from build123d import *

# Parameters (mm, degrees)
BOSS_EXTRUDE1_DEPTH = 111.8
SKETCH7_W           = 122.268
SKETCH7_H           = 249.395
BOSS_EXTRUDE2_DEPTH = 3
SKETCH8_W           = 9.0805
SKETCH8_H           = 57.785
BOSS_EXTRUDE3_DEPTH = 30
CUT_EXTRUDE1_DEPTH  = 9.0805
CUT_EXTRUDE2_DEPTH  = 9.0805
FILLET1_R           = 2


with BuildPart() as part:
    # Sketch6 → Boss-Extrude1 (new body)
    with BuildSketch(Plane(origin=(0, 0, 0), x_dir=(1, 0, 0), z_dir=(0, 1, 0))):
        Polygon((-809.2275, 2922.905), (-804.2275, 2922.905), (-804.2275, 2990.596), (-800.1, 2990.596), (-800.1, 3162.3), (-701.04, 3162.3), (-701.04, 3092.958), (-696.087, 3092.958), (-696.087, 2990.596), (-691.9595, 2990.596), (-691.9595, 2922.905), (-686.9595, 2922.905), (-686.9595, 3167.3), (-809.2275, 3167.3), align=None)
    extrude(amount=BOSS_EXTRUDE1_DEPTH)

    # Sketch7 → Boss-Extrude2 (add)
    with BuildSketch(Plane.XZ):
        with Locations((-748.0935, -3042.6025)):
            Rectangle(SKETCH7_W, SKETCH7_H)
    extrude(amount=BOSS_EXTRUDE2_DEPTH)

    # Sketch8 → Boss-Extrude3 (add)
    with BuildSketch(Plane(origin=(0, 0, 0), x_dir=(1, 0, 0), z_dir=(0, 1, 0))):
        with Locations((-795.55975, 3019.4885)):
            Rectangle(SKETCH8_W, SKETCH8_H)
        with Locations((-700.62725, 3019.4885)):
            Rectangle(SKETCH8_W, SKETCH8_H)
    extrude(amount=BOSS_EXTRUDE3_DEPTH)

    # Sketch9 → Cut-Extrude1 (cut)
    with BuildSketch(Plane(origin=(-791.0195, 0, 0), x_dir=(0, 0, -1), z_dir=(1, 0, 0))):
        Polygon((2990.596, 30), (2990.596, 15), (3005.596, 30), align=None)
        Polygon((3048.381, 30), (3033.381, 30), (3048.381, 15), align=None)
    extrude(amount=-CUT_EXTRUDE1_DEPTH, mode=Mode.SUBTRACT)

    # Sketch10 → Cut-Extrude2 (cut)
    with BuildSketch(Plane.ZY.offset(705.1675)):
        Polygon((-3048.381, 30), (-3048.381, 15), (-3033.381, 30), align=None)
        Polygon((-2990.596, 30), (-3005.596, 30), (-2990.596, 15), align=None)
    extrude(amount=-CUT_EXTRUDE2_DEPTH, mode=Mode.SUBTRACT)

    # Fillet1
    fillet1_edges = [part.edges().sort_by_distance(p)[0] for p in [
        (-809.2275, 55.9, -2922.905),
        (-809.2275, 54.4, -3167.3),
        (-686.9595, 54.4, -3167.3),
        (-686.9595, 55.9, -2922.905),
    ]]
    fillet(fillet1_edges, radius=FILLET1_R)


solid = part.part
Can you work these out from the model? Positions are in its coordinate system, mm. A direction names the side the tool comes from. Coordinates: 2 decimals unless noted, no trailing zeros. Write each loop counter-clockwise with the first axis right and the second up, starting at its lowest first coordinate (ties: lowest second). Pieces come first, ordered by that corner, then holes. Notation, with made-up numbers: M 4.5,83 L 36.5,83 A9 cw 36.5,93 Z; hole C -30,39 d1. An arc over 180 degrees is marked long. Use one line per item in the form item = value.
Q1. For P1, Ø2, axis at x = -702, z = -3049.5, coming from the +Y side; P2, Ø6.5, axis at x = -800, y = 55, coming from the +Z side; P3, Ø0.9, axis at x = -690.5, y = 63.5, coming from the +Z side (3 decimals), each with a flat end and sliding along its axis, tell me the tip position at first contact or that it passes through.
Model answer:
P1 = 0
P2 = -2990.6
P3 = -2922.905
Q2. If we section it at B-B (z = -3062): Write out the boundary of the cut face in (x, y), then the cut area to 3 significant figures.
Model answer:
outline = M -809.23,-3 L -686.96,-3 L -686.96,111.8 L -696.09,111.8 L -696.09,0 L -800.1,0 L -800.1,111.8 L -809.23,111.8 Z
area = 2,410 mm^2
Q3. If we section it at A-A (y = 35): Write out the boundary of the cut face in (x, z) (1 decimal), then the cut area to 3 significant figures.
Model answer:
outline = M -809.2,-3165.3 A2 ccw -807.2,-3167.3 L -689,-3167.3 A2 ccw -687,-3165.3 L -687,-2924.9 A2 ccw -689,-2922.9 L -692,-2922.9 L -692,-2990.6 L -696.1,-2990.6 L -696.1,-3093 L -701,-3093 L -701,-3162.3 L -800.1,-3162.3 L -800.1,-2990.6 L -804.2,-2990.6 L -804.2,-2922.9 L -807.2,-2922.9 A2 ccw -809.2,-2924.9 Z
area = 4,760 mm^2
Q4. For faces 4 (the flat face through (-795.5, 22.6, -3040.78)), 5 (the flat face through (-705.168, 15, -3019)), 6 (the flat face through (-749, -3, -3041)), which set-ups out of +Z, -Z, +X, -X, +Y, -Y let a thin tool reach every point of the face, with its end or its side?
Model answer:
face_4 = +Y
face_5 = +Z, +Y
face_6 = +Z, -Z, +X, -X, -Y
Q5. If we section it at D-D (y = 10): Write out the boundary of the cut face in (x, z) (1 decimal), then the cut area to 3 significant figures.
Model answer:
outline = M -809.2,-3165.3 A2 ccw -807.2,-3167.3 L -689,-3167.3 A2 ccw -687,-3165.3 L -687,-2924.9 A2 ccw -689,-2922.9 L -692,-2922.9 L -692,-2990.6 L -705.2,-2990.6 L -705.2,-3048.4 L -696.1,-3048.4 L -696.1,-3093 L -701,-3093 L -701,-3162.3 L -800.1,-3162.3 L -800.1,-3048.4 L -791,-3048.4 L -791,-2990.6 L -804.2,-2990.6 L -804.2,-2922.9 L -807.2,-2922.9 A2 ccw -809.2,-2924.9 Z
area = 5,810 mm^2
Q6. If we section it at C-C (x = -765): Write out the boundary of the cut face in (y, z) (3 decimals).
Model answer:
outline = M -3,-3167.3 L 111.8,-3167.3 L 111.8,-3162.3 L 0,-3162.3 L 0,-2917.905 L -3,-2917.905 Z
Q7. I need wall thicknesses on line 1 along X through (y, z) = (50, -2978); line 2 along X through (y, z) = (30, -3108); line 3 along Z through (x, y) = (-757, 33). Which ranges of each line are inside material? Lowest first, please. Write a range as from..to.
Model answer:
line_1 = -809.23..-804.23, -691.96..-686.96
line_2 = -809.23..-800.1, -701.04..-686.96
line_3 = -3167.3..-3162.3
Q8. We'd pull the mould along X, two halves only. Please class faces 1 (the flat face through (-809.228, 55, -3043)), 2 (the flat face through (-749, 55, -3167.3)), 3 (the flat face through (-701.04, 55, -3128)): +X half, -X half, draft (parallel to the pull), parting line (faces both ways), or undercut.
Model answer:
face_1 = -X half
face_2 = draft
face_3 = undercut
